Can you work these out from the model? Positions are in its coordinate system, mm. Round coordinates to 2 decimals unless told otherwise and drop trailing zeros. Loops run counter-clockwise (first coordinate to the right, second up) from the corner with the lowest first, then second, coordinate; pieces in that order, holes last.
(1) Thinking about a two-plate mould opening in Z: for faces 1 (the face through (22, 6.35, -71)), 2 (the face through (158.713, 3.131, -208.991)), which applies, released by +Z, released by -Z, zero draft, split by the parting line, or undercut?
(2) If I drill on line 1 along X through (y, z) = (6.25, -70.5); line 2 along X through (y, z) = (4.5, 71.5); line 3 along Z through (x, y) = (-15, 2.75), over which ranges is the centre line in solid material (lowest first)?
(3) Will these pins go through, and if not, where does the flat tip stop? pin 1 Ø4 at (x, z) = (129.5, 40) entering from -Y; pin 2 Ø1.8 at (x, z) = (149.41, -132.47) entering from -Y.
(4) I want a section at A-A on z = -63. Write out the boundary of the cut face in (x, y).
from build123d import *

# Parameters (mm, degrees)
SKETCH2_W           = 304.8
SKETCH2_H           = 304.8
SKETCH2_R           = 1
SKETCH2_R_2         = 1.75
SKETCH2_R_3         = 5
SKETCH2_R_4         = 1.016
BOSS_EXTRUDE1_DEPTH = 6.35
FILLET1_R           = 5
FILLET2_R           = 5
FILLET3_R           = 5
FILLET4_R           = 5


with BuildPart() as part:
    # Sketch2 → Boss-Extrude1 (new body)
    with BuildSketch(Plane(origin=(0, 0, 0), x_dir=(1, 0, 0), z_dir=(0, 1, 0))):
        with Locations((24.008323043, 69.071116712)):
            Rectangle(SKETCH2_W, SKETCH2_H)
        with Locations((-101.391676957, 132.471116712)):
            Circle(SKETCH2_R, mode=Mode.SUBTRACT)
        with Locations((-69.391676957, 132.471116712)):
            Circle(SKETCH2_R, mode=Mode.SUBTRACT)
        with Locations((-101.391676957, 194.471116712)):
            Circle(SKETCH2_R, mode=Mode.SUBTRACT)
        with Locations((-69.391676957, 194.471116712)):
            Circle(SKETCH2_R, mode=Mode.SUBTRACT)
        with Locations((149.408323043, 132.471116712)):
            Circle(SKETCH2_R, mode=Mode.SUBTRACT)
        with Locations((117.408323043, 132.471116712)):
            Circle(SKETCH2_R, mode=Mode.SUBTRACT)
        with Locations((117.408323043, 194.471116712)):
            Circle(SKETCH2_R, mode=Mode.SUBTRACT)
        with Locations((149.408323043, 194.471116712)):
            Circle(SKETCH2_R, mode=Mode.SUBTRACT)
        with Locations((114.958323043, 0.121116712)):
            Circle(SKETCH2_R_2, mode=Mode.SUBTRACT)
        with Locations((114.958323043, -14.378883288)):
            Circle(SKETCH2_R_2, mode=Mode.SUBTRACT)
        with Locations((-70.941676957, -1.996483288)):
            Circle(SKETCH2_R_2, mode=Mode.SUBTRACT)
        with Locations((-56.441676957, -1.996483288)):
            Circle(SKETCH2_R_2, mode=Mode.SUBTRACT)
        with Locations((163.708323043, 208.771116712)):
            Circle(SKETCH2_R_3, mode=Mode.SUBTRACT)
        with Locations((-115.691676957, 208.771116712)):
            Circle(SKETCH2_R_3, mode=Mode.SUBTRACT)
        with Locations((163.708323043, -70.628883288)):
            Circle(SKETCH2_R_3, mode=Mode.SUBTRACT)
        with Locations((-115.691676957, -70.628883288)):
            Circle(SKETCH2_R_3, mode=Mode.SUBTRACT)
        with Locations((43.439323043, -3.064883288)):
            Circle(SKETCH2_R_4, mode=Mode.SUBTRACT)
        with Locations((43.439323043, -51.324883288)):
            Circle(SKETCH2_R_4, mode=Mode.SUBTRACT)
        with Locations((-14.980676957, -3.064883288)):
            Circle(SKETCH2_R_4, mode=Mode.SUBTRACT)
        with Locations((-14.980676957, -51.324883288)):
            Circle(SKETCH2_R_4, mode=Mode.SUBTRACT)
        with BuildLine():
            Line((56.583323043, 54.371116712), (56.583323043, 79.771116712))
            ThreePointArc((56.583323043, 79.771116712), (53.383323043, 82.971116712), (50.183323043, 79.771116712))
            Line((50.183323043, 79.771116712), (50.183323043, 54.371116712))
            ThreePointArc((50.183323043, 54.371116712), (53.383323043, 51.171116712), (56.583323043, 54.371116712))
        make_face(mode=Mode.SUBTRACT)
        with BuildLine():
            Line((56.583323043, 157.571116712), (56.583323043, 132.171116712))
            ThreePointArc((56.583323043, 132.171116712), (53.383323043, 128.971116712), (50.183323043, 132.171116712))
            Line((50.183323043, 132.171116712), (50.183323043, 157.571116712))
            ThreePointArc((50.183323043, 157.571116712), (53.383323043, 160.771116712), (56.583323043, 157.571116712))
        make_face(mode=Mode.SUBTRACT)
        with BuildLine():
            Line((-8.566676957, 157.571116712), (-8.566676957, 132.171116712))
            ThreePointArc((-8.566676957, 132.171116712), (-5.366676957, 128.971116712), (-2.166676957, 132.171116712))
            Line((-2.166676957, 132.171116712), (-2.166676957, 157.571116712))
            ThreePointArc((-2.166676957, 157.571116712), (-5.366676957, 160.771116712), (-8.566676957, 157.571116712))
        make_face(mode=Mode.SUBTRACT)
        with BuildLine():
            Line((-8.566676957, 54.371116712), (-8.566676957, 79.771116712))
            ThreePointArc((-8.566676957, 79.771116712), (-5.366676957, 82.971116712), (-2.166676957, 79.771116712))
            Line((-2.166676957, 79.771116712), (-2.166676957, 54.371116712))
            ThreePointArc((-2.166676957, 54.371116712), (-5.366676957, 51.171116712), (-8.566676957, 54.371116712))
        make_face(mode=Mode.SUBTRACT)
    extrude(amount=BOSS_EXTRUDE1_DEPTH)

    # Fillet1
    fillet1_edges = [part.edges().sort_by_distance(p)[0] for p in [
        (176.408323043, 3.175, -221.471116712),
    ]]
    fillet(fillet1_edges, radius=FILLET1_R)

    # Fillet2
    fillet2_edges = [part.edges().sort_by_distance(p)[0] for p in [
        (-128.391676957, 3.175, -221.471116712),
    ]]
    fillet(fillet2_edges, radius=FILLET2_R)

    # Fillet3
    fillet3_edges = [part.edges().sort_by_distance(p)[0] for p in [
        (-128.391676957, 3.175, 83.328883288),
    ]]
    fillet(fillet3_edges, radius=FILLET3_R)

    # Fillet4
    fillet4_edges = [part.edges().sort_by_distance(p)[0] for p in [
        (176.408323043, 3.175, 83.328883288),
    ]]
    fillet(fillet4_edges, radius=FILLET4_R)


solid = part.part
Filled sheet:
1. face 1: zero draft
1. face 2: undercut
2. line 1: x = -128.39 to -8.57, -2.17 to 50.18, 56.58 to 176.41
2. line 2: x = -128.39 to -120.62, -110.77 to 158.78, 168.63 to 176.41
2. line 3: z = -221.47 to 2.05, 4.08 to 50.31, 52.34 to 83.33
3. pin 1: stops at y = 0
3. pin 2: passes through
4. outline: (-128.39, 0) - (-8.57, 0) - (-8.57, 6.35) - (-128.39, 6.35) - close; (-2.17, 0) - (50.18, 0) - (50.18, 6.35) - (-2.17, 6.35) - close; (56.58, 0) - (176.41, 0) - (176.41, 6.35) - (56.58, 6.35) - close
